from build123d import *

# Parameters (mm, degrees)
F0_W     = 78.1559348106
F0_H     = 11.1243845895
F1_DEPTH = 25.4
F0_R     = 9.006561322
F2_DEPTH = 12.7
F3_R     = 12.7
F4_R     = 3.4818048238
F5_DEPTH = 11.1253845895


# Not quite as in the source:
# - ends of sketch curves that miss each other by under 0.0002 mm in the source are joined


with BuildPart() as f1:
    # F0 (on Top) → F1 (new body)
    with BuildSketch(Plane.XY):
        Rectangle(F0_W, F0_H)
    extrude(amount=F1_DEPTH)



with BuildPart() as f1b:
    # F0 (on Top) → F1, piece 2 (new body)
    with BuildSketch(Plane.XY):
        with BuildLine():
            Line((-16.3389042508, 50.9063668795), (-16.3389042508, 49.7835881762))
            ThreePointArc((-16.3389042508, 49.7835881762), (-0.5764210141, 34.0065966737), (16.2587184459, 48.6335381866))
            ThreePointArc((16.2587184459, 48.6335381866), (1.1371213689, 66.6539292144), (-16.3389042508, 50.9063668795))
        make_face()
        with Locations((0, 50.3449775279)):
            Circle(F0_R, mode=Mode.SUBTRACT)
    extrude(amount=F1_DEPTH)


with BuildPart() as f1_1:
    add(f1.part)

    add(f1b.part)  # F2 merges F1b
    # F0 (on Top) → F2 (join)
    with BuildSketch(Plane.XY):
        with BuildLine():
            ThreePointArc((-16.3389042508, 28.4221922947), (-23.0344432329, 12.2577312768), (-39.1989042508, 5.5621922947))
            Line((-39.1989042508, 5.5621922947), (-39.0779674053, 5.5621922947))
            Line((-39.0779674053, 5.5621922947), (39.0779674053, 5.5621922947))
            ThreePointArc((39.0779674053, 5.5621922947), (22.9398561975, 12.2721453491), (16.2587184459, 28.4221922947))
            Line((16.2587184459, 28.4221922947), (16.2587184459, 48.6335381866))
            ThreePointArc((16.2587184459, 48.6335381866), (-0.5764210141, 34.0065966737), (-16.3389042508, 49.7835881762))
            Line((-16.3389042508, 49.7835881762), (-16.3389042508, 28.4221922947))
        make_face()
    extrude(amount=F2_DEPTH)

    # F3
    f3_edges = [f1_1.edges().sort_by_distance(p)[0] for p in [
        (39.077967, 0, 25.4),
        (-39.077967, 0, 25.4),
    ]]
    fillet(f3_edges, radius=F3_R)

    # F4 (on face) → F5 (cut, through all)
    with BuildSketch(Plane(origin=(0, 5.5621922947, 0), x_dir=(-1, 0, 0), z_dir=(0, 1, 0))):
        with Locations((-26.2421388179, 19.2537438124)):
            Circle(F4_R)
        with Locations((26.2421388179, 19.2537438124)):
            Circle(F4_R)
    extrude(amount=-F5_DEPTH, mode=Mode.SUBTRACT)


solid = f1_1.part
Verification items for the finished model (mm, model axes). A direction names the side the tool comes from. Give positions to 0.01 mm unless a question says otherwise; leave off trailing zeros. Write each loop counter-clockwise with the first axis right and the second up, starting at its lowest first coordinate (ties: lowest second). Pieces come first, ordered by that corner, then holes. Notation, with made-up numbers: M 56.25,78 L 60.25,78 A22 cw 60.25,104 Z; hole C 69,-21.75 d9. An arc over 180 degrees is marked long. Put each result on its own line as item: value. Start each with the question number.
1. Section check A-A (x = 0). Record the cut outline in (y, z).
2. Section check C-C (z = 9.75). Record the cut outline in (x, y), and give its area (3 significant figures).
3. Scan lines: line 1 along Y through (x, z) = (-3, 16.5); line 2 along X through (y, z) = (33, 2.75); line 3 along X through (y, z) = (42, 23). Record each from-to range of solid material in increasing order. Write a range as [from, to].
4. Section check B-B (y = 42.5). Record the cut outline in (x, z).
5. Go/stop test with flat-tipped pins: pin 1 Ø2 at (y, z) = (24, 7.5) entering from -X; pin 2 Ø10 at (y, z) = (35.5, 4.5) entering from +X; pin 3 Ø10 at (x, y) = (21, 14) entering from +Z. Record where each tip stops, or that it passes through.
6. Section check D-D (y = 32.5). Record the cut outline in (x, z), and give its area (3 significant figures).
7. Draft check along Z on faces 4 (the face through (25, 0, 16)), 5 (the face through (0, 0, 25.4)), 6 (the face through (-1, 5.562, 19)). Enter one of: +Z half, -Z half, draft (parallel to the pull), parting line (faces both ways), or undercut.
8. Set-up check for faces 1 (the face through (-16.339, 40, 7)), 2 (the face through (16.259, 38, 6)), 3 (the face through (3.78, 66.25, 15.34)): record each of +Z, -Z, +X, -X, +Y, -Y from which the full face is reachable in a straight line by a thin tool's end or side.
Answer list:
1. outline: M -5.56,0 L 41.34,0 L 41.34,25.4 L 34,25.4 L 34,12.7 L 5.56,12.7 L 5.56,25.4 L -5.56,25.4 Z; M 59.35,0 L 66.69,0 L 66.69,25.4 L 59.35,25.4 Z
2. outline: M -39.2,5.56 L -39.08,5.56 L -39.08,-5.56 L 39.08,-5.56 L 39.08,5.56 A22.86 cw 16.26,28.42 L 16.26,48.63 A16.35 ccw long -16.34,50.91 L -16.34,28.42 A22.86 cw Z; hole C 0,50.34 d18.01
2. area: 2,720 mm2
3. line 1: [-5.56, 5.56], [34.27, 41.85], [58.84, 66.42]
3. line 2: [-16.34, 16.26]
3. line 3: [-14.06, -3.39], [3.39, 14.06]
4. outline: M -16.34,0 L -4.42,0 L -4.42,25.4 L -14.34,25.4 L -14.34,12.7 L -16.34,12.7 Z; M 4.42,0 L 16.26,0 L 16.26,12.7 L 14.34,12.7 L 14.34,25.4 L 4.42,25.4 Z
5. pin 1: x = -16.99
5. pin 2: x = 16.26
5. pin 3: z = 12.7
6. outline: M -16.34,0 L 16.26,0 L 16.26,12.7 L -16.34,12.7 Z
6. area: 414 mm2
7. face 4: undercut
7. face 5: +Z half
7. face 6: draft
8. face 1: +Z, -Z, -X, +Y
8. face 2: +Z, -Z, +X
8. face 3: +Z
